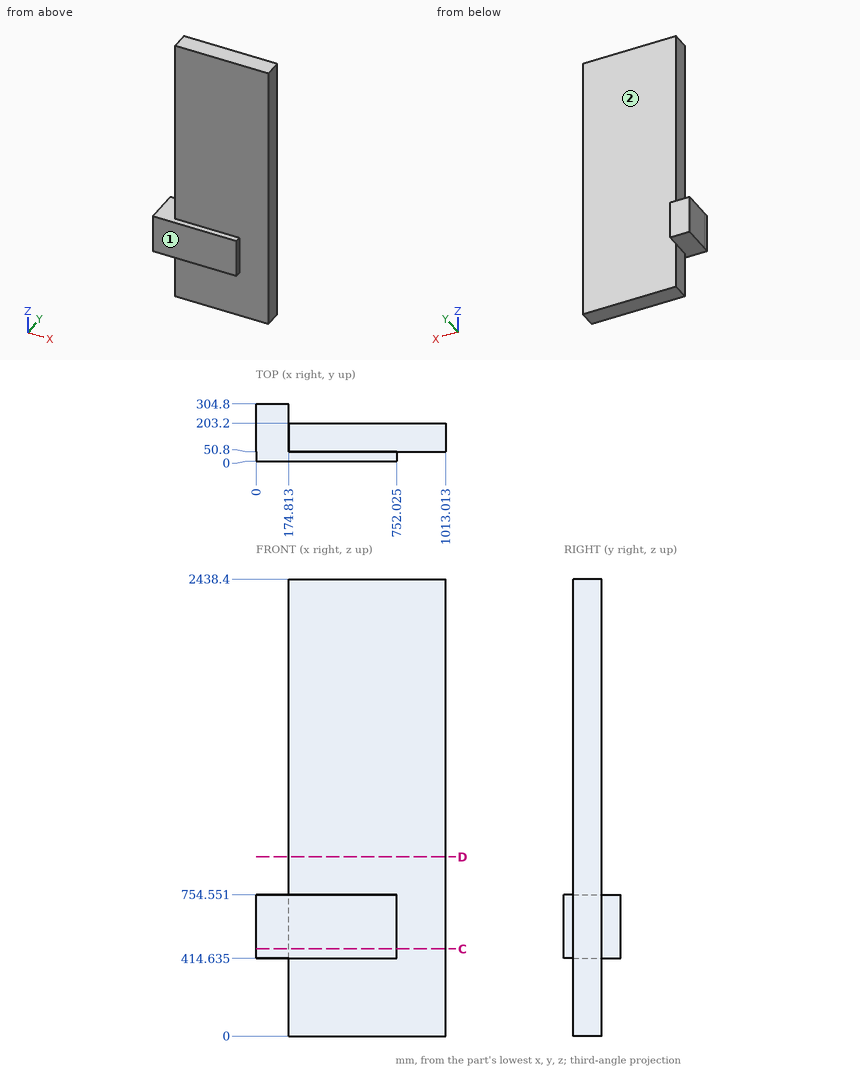
For this review, use the dimensioned drawing (mm, ordinates from the lowest corner) and the shaded views. A direction names the side the tool comes from. Coordinates: 2 decimals unless noted, no trailing zeros. Loops run counter-clockwise (first coordinate to the right, second up) from the corner with the lowest first, then second, coordinate; pieces in that order, holes last. Notation, with made-up numbers: (25.5, 78.25) -> (59.5, 78.25) arc R15 ccw to (59.5, 92.25) -> close; hole circle Ø6 at (82.25, 15.5). An arc over 180 degrees is marked (long way). Use a Markdown table: item, result. Add a question column.
Item 1: We need section C-C, the plane z = 465. Write out the cut boundary in (x, y) (1 decimal), and give its area (3 significant figures).
Item 2: Clearance check with flat-ended pins moving along their axes: P1, Ø10, axis at x = 264.5, z = 1708, coming from the +Y side; P2, Ø3, axis at y = 198.5, z = 898.5, coming from the -X side. State where each tip first meets the part, or that it passes through.
Item 3: Wall thickness on L1, parallel to Y at x = 927, z = 2297; L2, parallel to X at y = 112.5, z = 992; L3, parallel to Y at x = 654, z = 690: over which ranges is each line inside the solid? List them lowest first. Write a range as from..to.
Item 4: We need section D-D, the plane z = 955.5. Write out the cut boundary in (x, y).
Item 5: Machinability: for the marked faces 1 and 2, which of the approach directions +Z, -Z, +X, -X, +Y, -Y give a long, thin tool a straight path to every point of the face, cutting with its end or side? Answer none if there is none.
Numbers:
| question | item | result |
|---|---|---|
| 1 | outline | (0, 0) -> (752, 0) -> (752, 50.8) -> (1013, 50.8) -> (1013, 203.2) -> (174.8, 203.2) -> (174.8, 304.8) -> (0, 304.8) -> close |
| 1 | area | 210,000 mm^2 |
| 2 | P1 | stops at y = 203.2 |
| 2 | P2 | stops at x = 174.81 |
| 3 | L1 | y = 50.8..203.2 |
| 3 | L2 | x = 174.81..1013.01 |
| 3 | L3 | y = 0..203.2 |
| 4 | outline | (174.81, 50.8) -> (1013.01, 50.8) -> (1013.01, 203.2) -> (174.81, 203.2) -> close |
| 5 | face 1 | +Z, -Z, +X, -X, -Y |
| 5 | face 2 | +Z, -Z, +X, +Y |
